Autodesk Inventor part; units mm, degrees
ref_plane "YZ Plane" through (0, 0, 0) normal (1, 0, 0) x (0, 1, 0)
ref_plane "XZ Plane" through (0, 0, 0) normal (0, 1, 0) x (-1, 0, 0)
ref_plane "XY Plane" through (0, 0, 0) normal (0, 0, 1) x (1, 0, 0)
sketch "Sketch1" plane through (0, 0, 0) normal (0, 0, 1) x (1, 0, 0)
  line L0 (-17.5, 0) -> (17.5, 0) construction
  line L1 (0, -37.52) -> (0, 37.52) construction
  line L2 (-12.5, 26.8) -> (12.5, 26.8)
  line L3 (12.5, 26.8) -> (12.5, -26.8)
  line L4 (12.5, -26.8) -> (-12.5, -26.8)
  line L5 (-12.5, -26.8) -> (-12.5, 26.8)
  line L6 (-10.25, 23.3) -> (10.25, 23.3)
  line L7 (10.25, 23.3) -> (10.25, -23.3)
  line L8 (10.25, -23.3) -> (-10.25, -23.3)
  line L9 (-10.25, -23.3) -> (-10.25, 23.3)
  point P0 (0, 0)
  dimension "d0" = 20.5
  dimension "d1" = 25
  dimension "d3" = 46.6
  dimension "d8" = 3.5
  dimension "d9" = 3.5
  dimension "d10" = 53.6
extrude "Extrusion1" add sketch "Sketch1" along normal blind 3
properties part number "20_Cube_Insert_Sample_clamp"
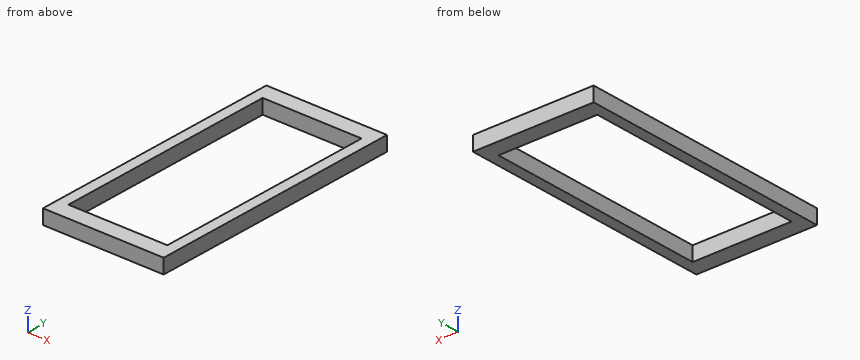
Read the model definition and answer for the solid it produces. Units are mm, in the model's axes. Round coordinates to 2 decimals unless told otherwise and drop trailing zeros. Loops run counter-clockwise (first coordinate to the right, second up) from the corner with the lowest first, then second, coordinate; pieces in that order, holes last.
Q1. Consider probe 1 along X at (y, z) = (22, 2.05); probe 2 along Y at (x, z) = (-7.25, 0.4). Determine where each line is inside the solid, lowest interval first.
Q2. Section B-B on x = 3.5 is taken. Write down the section's boundary in (y, z), and give its area (3 significant figures).
Q3. Section A-A on y = -13 is taken. Write down the section's boundary in (x, z).
Q4. Section C-C on z = 1.25 is taken. Write down the section's boundary in (x, y).
Q5. This flat-tipped pin is pushed along its axis until it touches: pin 1 (6 mm diameter, centred on x = -9.5, y = 17.5, fed in from +Z). Where does it stop, or does it pass through?
Output:
1. probe 1: x = -12.5 to -10.25, 10.25 to 12.5
1. probe 2: y = -26.8 to -23.3, 23.3 to 26.8
2. outline: (-26.8, 0) - (-23.3, 0) - (-23.3, 3) - (-26.8, 3) - close; (23.3, 0) - (26.8, 0) - (26.8, 3) - (23.3, 3) - close
2. area: 21.0 mm2
3. outline: (-12.5, 0) - (-10.25, 0) - (-10.25, 3) - (-12.5, 3) - close; (10.25, 0) - (12.5, 0) - (12.5, 3) - (10.25, 3) - close
4. outline: (-12.5, -26.8) - (12.5, -26.8) - (12.5, 26.8) - (-12.5, 26.8) - close; hole (-10.25, -23.3) - (10.25, -23.3) - (10.25, 23.3) - (-10.25, 23.3) - close
5. pin 1: stops at z = 3
